Geometry: final body of the model. Coordinates: model frame, mm. Face numbers are marked on the shaded views. A direction names the side the tool comes from. Give positions to 0.01 mm unless a question says otherwise; leave off trailing zeros. Loops run counter-clockwise (first coordinate to the right, second up) from the corner with the lowest first, then second, coordinate; pieces in that order, holes last. Notation, with made-up numbers: (43, 21.25) -> (80, 21.25) arc R27 ccw to (80, 37.25) -> close; hole circle Ø9 at (-24, 52). An arc over 180 degrees is marked (long way). Answer in a Markdown table with one row per item. Add a question column.
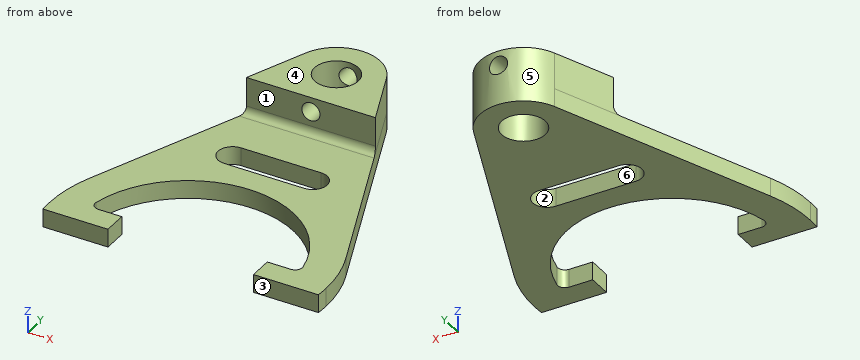
from build123d import *

# Parameters (mm, degrees)
ESTRUSIONE_ESTRUSIONE1_DEPTH = 5
ESTRUSIONE_ESTRUSIONE2_DEPTH = 10
RACCORDO1_R                  = 2
FORO_12_0_12_1_D             = 12
FORO_5_0_5_2_D               = 5
TAGLIO_ESTRUSIONE1_REACH     = 85.124


with BuildPart() as part:
    # Schizzo2 → Estrusione-Estrusione1 (new body)
    with BuildSketch(Plane.XY):
        with BuildLine():
            ThreePointArc((11.141538384, 4.457142857), (0, 12), (-11.141538384, 4.457142857))
            Line((-11.141538384, 4.457142857), (-35.281538214, -55.885714286))
            ThreePointArc((-35.281538214, -55.885714286), (-37.314196039, -62.813152713), (-38, -70))
            ThreePointArc((-38, -70), (-37.965175205, -71.626490584), (-37.860764652, -73.25))
            Line((-37.860764652, -73.25), (-20, -73.25))
            Line((-20, -73.25), (-20, -66.75))
            Line((-20, -66.75), (-28.817312505, -66.75))
            ThreePointArc((-28.817312505, -66.75), (0, -41), (28.817312505, -66.75))
            Line((28.817312505, -66.75), (20, -66.75))
            Line((20, -66.75), (20, -73.25))
            Line((20, -73.25), (37.860764652, -73.25))
            ThreePointArc((37.860764652, -73.25), (37.965175205, -71.626490584), (38, -70))
            ThreePointArc((38, -70), (37.314196039, -62.813152713), (35.281538214, -55.885714286))
            Line((35.281538214, -55.885714286), (11.141538384, 4.457142857))
        make_face()
    extrude(amount=ESTRUSIONE_ESTRUSIONE1_DEPTH)

    # Schizzo3 → Estrusione-Estrusione2 (add)
    with BuildSketch(Plane.XY.offset(5)):
        with BuildLine():
            Line((-17.725174701, -12), (17.725174701, -12))
            Line((17.725174701, -12), (11.141538384, 4.457142857))
            ThreePointArc((11.141538384, 4.457142857), (0, 12), (-11.141538384, 4.457142857))
            Line((-11.141538384, 4.457142857), (-17.725174701, -12))
        make_face()
    extrude(amount=ESTRUSIONE_ESTRUSIONE2_DEPTH)

    # Raccordo1
    raccordo1_edges = [part.edges().sort_by_distance(p)[0] for p in [
        (-28.817312505, -66.75, 2.5),
        (28.817312505, -66.75, 2.5),
        (0, -12, 5),
    ]]
    fillet(raccordo1_edges, radius=RACCORDO1_R)

    # Foro Ø12.0 (12)-1 (through all)
    with Locations(Plane.XY.offset(15)):
        with Locations((0, 0)):
            Hole(FORO_12_0_12_1_D / 2)

    # Foro Ø5.0 (5)-2 (through all)
    with Locations(Plane(origin=(0, -12, 0), x_dir=(-1, 0, 0), z_dir=(0, -1, 0))):
        with Locations((0, -11)):
            Hole(FORO_5_0_5_2_D / 2)

    # Schizzo8 → Taglio-Estrusione1 (cut, up to next)
    with BuildSketch(Plane.XY.offset(5), mode=Mode.PRIVATE) as taglio_estrusione1_sk1:
        with BuildLine():
            Line((-11, -26), (11, -26))
            ThreePointArc((11, -26), (15, -30), (11, -34))
            Line((11, -34), (-11, -34))
            ThreePointArc((-11, -34), (-15, -30), (-11, -26))
        make_face()
    taglio_estrusione1_tool1 = extrude(taglio_estrusione1_sk1.sketch, amount=-TAGLIO_ESTRUSIONE1_REACH, mode=Mode.PRIVATE) & part.part
    add(taglio_estrusione1_tool1.solids().sort_by_distance((0, -30, 5))[0], mode=Mode.SUBTRACT)


solid = part.part
(1) Reachability of the marked faces 1, 2 and 3 from +Z, -Z, +X, -X, +Y, -Y: full face, straight path, thin tool, end or side. Return the list, or none.
(2) Material intervals for line 1 along Z through (x, y) = (0, 9); line 2 along Z through (x, y) = (30, -66.5); line 3 along X through (y, z) = (-27, 3.25), sorted ascending. Write a range as from..to.
(3) Cut plane D-D on z = 3.25. Return the cut outline in (x, y), then the cut area to 3 significant figures.
(4) Cut plane C-C on z = 11. Return the cut outline in (x, y), then the cut area to 3 significant figures.
(5) Pin query (flat end, axial travel): pin 1 Ø3 at (y, z) = (-36, 6) entering from -X; pin 2 Ø2.5 at (x, z) = (-22.5, 1.5) entering from +Y; pin 3 Ø2.5 at (x, z) = (4.5, 2) entering from -Y; pin 4 Ø4 at (x, z) = (0, 11) entering from -Y. Return the tip coordinate at first contact, or that it passes through.
(6) Draft query along X for the marked faces 4, 5 and 6. Return one class per face: +X half, -X half, draft (parallel to the pull), parting line (faces both ways), or undercut.
(7) Cut plane B-B on y = -30. Return the cut outline in (x, z), then the cut area to 3 significant figures.
(8) Cut plane A-A on x = 0. Return the cut outline in (y, z).
Answer list:
| question | item | result |
|---|---|---|
| 1 | face 1 | +Z, +X, -X, -Y |
| 1 | face 2 | +Z, -Z |
| 1 | face 3 | +Z, -Z, +X, -X, -Y |
| 2 | line 1 | z = 0..8.5, 13.5..15 |
| 2 | line 2 | z = 0..5 |
| 2 | line 3 | x = -23.73..-13.65, 13.65..23.73 |
| 3 | outline | (-37.86, -73.25) -> (-20, -73.25) -> (-20, -66.75) -> (-26.48, -66.75) arc R2 cw to (-28.45, -64.36) arc R29 cw to (28.45, -64.36) arc R2 cw to (26.48, -66.75) -> (20, -66.75) -> (20, -73.25) -> (37.86, -73.25) arc R38 ccw to (35.28, -55.89) -> (11.14, 4.46) arc R12 ccw to (-11.14, 4.46) -> (-35.28, -55.89) arc R38 ccw to start; hole (-11, -34) -> (11, -34) arc R4 ccw to (11, -26) -> (-11, -26) arc R4 ccw to start; hole circle Ø12 at (0, 0) |
| 3 | area | 2,490 mm² |
| 4 | outline | (-17.73, -12) -> (-2.5, -12) -> (-2.5, -5.45) arc R6 cw to (-2.5, 5.45) -> (-2.5, 11.74) arc R12 ccw to (-11.14, 4.46) -> close; (2.5, -12) -> (17.73, -12) -> (11.14, 4.46) arc R12 ccw to (2.5, 11.74) -> (2.5, 5.45) arc R6 cw to (2.5, -5.45) -> close |
| 4 | area | 422 mm² |
| 5 | pin 1 | stops at x = -27.77 |
| 5 | pin 2 | stops at y = -20.81 |
| 5 | pin 3 | stops at y = -41.58 |
| 5 | pin 4 | passes through |
| 6 | face 4 | draft |
| 6 | face 5 | parting line |
| 6 | face 6 | undercut |
| 7 | outline | (-24.93, 0) -> (-15, 0) -> (-15, 5) -> (-24.93, 5) -> close; (15, 0) -> (24.93, 0) -> (24.93, 5) -> (15, 5) -> close |
| 7 | area | 99.3 mm² |
| 8 | outline | (-41, 0) -> (-34, 0) -> (-34, 5) -> (-41, 5) -> close; (-26, 0) -> (-6, 0) -> (-6, 8.5) -> (-12, 8.5) -> (-12, 7) arc R2 cw to (-14, 5) -> (-26, 5) -> close; (-12, 13.5) -> (-6, 13.5) -> (-6, 15) -> (-12, 15) -> close; (6, 0) -> (12, 0) -> (12, 8.5) -> (6, 8.5) -> close; (6, 13.5) -> (12, 13.5) -> (12, 15) -> (6, 15) -> close |
